Model file for the job. Use its own axes, mm. Face numbers are marked on the shaded views. A direction names the side the tool comes from. Round coordinates to 2 decimals unless told otherwise and drop trailing zeros. Loops run counter-clockwise (first coordinate to the right, second up) from the corner with the lowest first, then second, coordinate; pieces in that order, holes last. Notation, with made-up numbers: M -14,-28.5 L 20,-28.5 A13 ccw 20,-22.5 Z; hole C 77,29.25 d7. An arc over 180 degrees is marked long. Use a Markdown table: item, result. Add a question column.
Item 1: Saw through at C-C on x = 58. Write the cut outline in (y, z) (3 decimals), then the cut area to 3 significant figures.
Item 2: Wall check: L1, parallel to Z at x = 91, y = -41 (3 decimals); L2, parallel to Y at x = -12, z = 33; L3, parallel to X at y = -1, z = 1.5 (3 decimals). Give the ranges that are in metal, low to high. Write a range as from..to.
Item 3: Tool access for the marked faces 1, 2, 3 and 4: list every direction of +Z, -Z, +X, -X, +Y, -Y with a clear straight run to the whole face (end or side of a thin tool).
Item 4: Saw through at A-A on y = 28.5. Write the cut outline in (x, z) (3 decimals), then the cut area to 3 significant figures.
Item 5: Saw through at B-B on z = 5. Write the cut outline in (x, y) (3 decimals).
Item 6: Pin check, flat tips, straight feed: P1, Ø18.5, axis at y = 2, z = 14, coming from the +X side (3 decimals); P2, Ø16.5, axis at x = 10.5, y = -35.5, coming from the +Z side (3 decimals); P3, Ø15.5, axis at x = 8.5, z = 47, coming from the -Y side. Stop position of each tip, or through.
```python
from build123d import *

# Parameters (mm, degrees)
F1_DEPTH = 63.5
F0_W     = 4.859683
F0_H     = 4.7752
F2_DEPTH = 25.4
F3_DEPTH = 7.9375


with BuildPart() as f1:
    # F0 (on Front) → F1 (new body, symmetric)
    with BuildSketch(Plane.XZ):
        Polygon((-41.275, 9.525), (-41.275, -9.525), (41.275, -9.525), (41.275, 9.525), (22.225, 9.525), align=None)
    extrude(amount=F1_DEPTH, both=True)

    # F0 (on Front) → F2 (join, symmetric)
    with BuildSketch(Plane.XZ):
        with BuildLine():
            Line((22.225, 9.525), (41.275, 9.525))
            Line((41.275, 9.525), (41.275, 27.0002))
            ThreePointArc((41.275, 27.0002), (45.92468, 38.22552), (57.15, 42.8752))
            Line((57.15, 42.8752), (80.865317, 42.8752))
            Line((80.865317, 42.8752), (80.865317, 61.9252))
            Line((80.865317, 61.9252), (57.15, 61.9252))
            ThreePointArc((57.15, 61.9252), (32.454296, 51.695904), (22.225, 27.0002))
            Line((22.225, 27.0002), (22.225, 9.525))
        make_face()
        with Locations((83.295158, 40.4876)):
            Rectangle(F0_W, F0_H)
    extrude(amount=F2_DEPTH, both=True)

    # F0 (on Front) → F3 (join, symmetric)
    with BuildSketch(Plane.XZ):
        with BuildLine():
            add(Edge.make_bspline(
                [(-41.275, 9.525), (-41.275, 31.890627), (15.217554, 61.9252), (57.15, 61.9252)],
                knots=[0, 0, 0, 0, 111.504536, 111.504536, 111.504536, 111.504536], degree=3))
            Line((-41.275, 9.525), (22.225, 9.525))
            Line((22.225, 9.525), (22.225, 27.0002))
            ThreePointArc((22.225, 27.0002), (32.454296, 51.695904), (57.15, 61.9252))
        make_face()
    extrude(amount=F3_DEPTH, both=True)

    # F0 (on Front) → F4 (revolve)
    with BuildSketch(Plane.XZ):
        Polygon((85.725, 66.675), (85.725, 61.9252), (85.725, 42.8752), (85.725, 38.1), (131.665317, 38.1), (131.665317, 66.675), align=None)
    revolve(axis=Axis((85.725, 0, 52.3875), (0, 0, 1)))


solid = f1.part
```
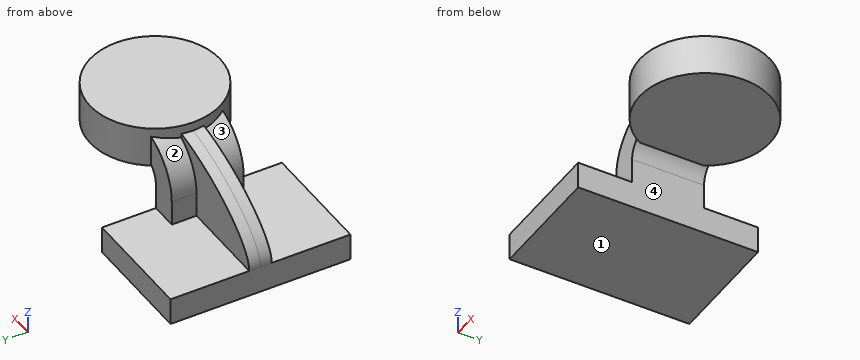
Entries:
| question | item | result |
|---|---|---|
| 1 | outline | M -36.631,38.1 L 36.631,38.1 L 36.631,66.675 L -36.631,66.675 Z |
| 1 | area | 2,090 mm2 |
| 2 | L1 | 38.1..66.675 |
| 2 | L2 | -7.94..7.94 |
| 2 | L3 | -41.275..41.275 |
| 3 | face 1 | -Z, +X, -X, +Y, -Y |
| 3 | face 2 | +Z, -X, +Y |
| 3 | face 3 | +Z, -X, -Y |
| 3 | face 4 | -Z, +X, +Y, -Y |
| 4 | outline | M -41.275,-9.525 L 41.275,-9.525 L 41.275,9.525 L -41.275,9.525 Z; M 49.694,38.1 L 121.756,38.1 L 121.756,66.675 L 49.694,66.675 Z |
| 4 | area | 3,630 mm2 |
| 5 | outline | M -41.275,-63.5 L 41.275,-63.5 L 41.275,63.5 L -41.275,63.5 Z |
| 6 | P1 | x = 41.275 |
| 6 | P2 | z = 9.525 |
| 6 | P3 | y = -7.94 |
